```python
from build123d import *

# Parameters (mm, degrees)
SKETCH_1_W             = 160
SKETCH_1_H             = 124
EXTRUDE_1_DEPTH        = 3
SKETCH_2_R             = 1.5
CUT_EXTRUDE_1_DEPTH    = 10
SKETCH_3_R             = 2
CUT_EXTRUDE_2_DEPTH    = 172.618763543
SKETCH_4_R             = 1.5
CUT_EXTRUDE_3_DEPTH    = 10
PATTERN_LINEAR_1_COUNT = 7
PATTERN_LINEAR_1_PITCH = 8
SKETCH_6_R             = 1.5
CUT_EXTRUDE_4_DEPTH    = 10
SKETCH_7_R             = 1.5
CUT_EXTRUDE_5_DEPTH    = 10
SKETCH_8_R             = 1.5
CUT_EXTRUDE_6_DEPTH    = 10
SKETCH_9_R             = 1.5
CUT_EXTRUDE_7_DEPTH    = 10
SKETCH_10_R            = 4
CUT_EXTRUDE_8_DEPTH    = 10
FILLET_1_R             = 2
SKETCH_12_R            = 1.5
CUT_EXTRUDE_10_DEPTH   = 10
SKETCH_13_R            = 1.75
CUT_EXTRUDE_11_DEPTH   = 70
SKETCH_14_R            = 1.5
CUT_EXTRUDE_12_DEPTH   = 4
SKETCH_15_R            = 2.5
CUT_EXTRUDE_13_DEPTH   = 10


with BuildPart() as part:
    # 草圖1 → 填料-伸長1 (new body)
    with BuildSketch(Plane(origin=(0, 0, 0), x_dir=(1, 0, 0), z_dir=(0, 1, 0))):
        with Locations((80, 0)):
            Rectangle(SKETCH_1_W, SKETCH_1_H)
    extrude(amount=EXTRUDE_1_DEPTH)

    # 草圖2 → 除料-伸長1 (cut)
    with BuildSketch(Plane(origin=(0, 3, 0), x_dir=(1, 0, 0), z_dir=(0, 1, 0))):
        with Locations(Location((113, 52, 0), (0, 0, 270))):
            Circle(SKETCH_2_R)
        with Locations(Location((130, 52, 0), (0, 0, 270))):
            Circle(SKETCH_2_R)
        with Locations(Location((113, -52, 0), (0, 0, 270))):
            Circle(SKETCH_2_R)
        with Locations(Location((130, -52, 0), (0, 0, 270))):
            Circle(SKETCH_2_R)
    extrude(amount=-CUT_EXTRUDE_1_DEPTH, mode=Mode.SUBTRACT)

    # 草圖3 → 除料-伸長2 (cut, through all)
    with BuildSketch(Plane.XZ):
        with Locations(Location((25, 19.5, 0), (0, 0, 270))):
            Circle(SKETCH_3_R)
        with Locations(Location((25, -19.5, 0), (0, 0, 270))):
            Circle(SKETCH_3_R)
    extrude(amount=-CUT_EXTRUDE_2_DEPTH, mode=Mode.SUBTRACT)

    # 草圖4 → 除料-伸長3 (cut)
    with BuildSketch(Plane(origin=(0, 3, 0), x_dir=(1, 0, 0), z_dir=(0, 1, 0))):
        with Locations(Location((5, 24, 0), (0, 0, 270))):
            Circle(SKETCH_4_R)
    cut_extrude_3 = extrude(amount=-CUT_EXTRUDE_3_DEPTH, mode=Mode.SUBTRACT)

    # 直線複製排列1: 除料-伸長3 ×7
    with Locations(*[(0, 0, i * PATTERN_LINEAR_1_PITCH) for i in range(1, PATTERN_LINEAR_1_COUNT)]):
        add(cut_extrude_3, mode=Mode.SUBTRACT)

    # 草圖6 → 除料-伸長4 (cut)
    with BuildSketch(Plane(origin=(0, 3, 0), x_dir=(1, 0, 0), z_dir=(0, 1, 0))):
        with Locations(Location((100, 19, 0), (0, 0, 270))):
            Circle(SKETCH_6_R)
        with Locations(Location((137, 19, 0), (0, 0, 270))):
            Circle(SKETCH_6_R)
        with Locations(Location((100, -18, 0), (0, 0, 270))):
            Circle(SKETCH_6_R)
        with Locations(Location((137, -18, 0), (0, 0, 270))):
            Circle(SKETCH_6_R)
    extrude(amount=-CUT_EXTRUDE_4_DEPTH, mode=Mode.SUBTRACT)

    # 草圖7 → 除料-伸長5 (cut)
    with BuildSketch(Plane(origin=(0, 3, 0), x_dir=(1, 0, 0), z_dir=(0, 1, 0))):
        with Locations(Location((49.8, 30.6, 0), (0, 0, 270))):
            Circle(SKETCH_7_R)
        with Locations(Location((77.8, 30.6, 0), (0, 0, 270))):
            Circle(SKETCH_7_R)
        with Locations(Location((34.6, -20.4, 0), (0, 0, 270))):
            Circle(SKETCH_7_R)
        with Locations(Location((82.6, -21, 0), (0, 0, 270))):
            Circle(SKETCH_7_R)
    extrude(amount=-CUT_EXTRUDE_5_DEPTH, mode=Mode.SUBTRACT)

    # 草圖8 → 除料-伸長6 (cut)
    with BuildSketch(Plane(origin=(0, 3, 0), x_dir=(1, 0, 0), z_dir=(0, 1, 0))):
        with Locations(Location((37, 52, 0), (0, 0, 270))):
            Circle(SKETCH_8_R)
        with Locations(Location((145, 52, 0), (0, 0, 270))):
            Circle(SKETCH_8_R)
        with Locations(Location((37, -52, 0), (0, 0, 270))):
            Circle(SKETCH_8_R)
        with Locations(Location((145, -52, 0), (0, 0, 270))):
            Circle(SKETCH_8_R)
    extrude(amount=-CUT_EXTRUDE_6_DEPTH, mode=Mode.SUBTRACT)

    # 草圖9 → 除料-伸長7 (cut)
    with BuildSketch(Plane(origin=(0, 3, 0), x_dir=(1, 0, 0), z_dir=(0, 1, 0))):
        with Locations(Location((91, -52, 0), (0, 0, 270))):
            Circle(SKETCH_9_R)
        with Locations(Location((91, 52, 0), (0, 0, 270))):
            Circle(SKETCH_9_R)
    extrude(amount=-CUT_EXTRUDE_7_DEPTH, mode=Mode.SUBTRACT)

    # 草圖10 → 除料-伸長8 (cut)
    with BuildSketch(Plane(origin=(0, 3, 0), x_dir=(1, 0, 0), z_dir=(0, 1, 0))):
        with Locations(Location((25, 37, 0), (0, 0, 270))):
            Circle(SKETCH_10_R)
        with Locations(Location((25, -37, 0), (0, 0, 270))):
            Circle(SKETCH_10_R)
    extrude(amount=-CUT_EXTRUDE_8_DEPTH, mode=Mode.SUBTRACT)

    # 圓角1
    fillet_1_edges = [part.edges().sort_by_distance(p)[0] for p in [
        (160, 1.5, -62),
        (160, 1.5, 62),
    ]]
    fillet(fillet_1_edges, radius=FILLET_1_R)

    # 草圖12 → 除料-伸長10 (cut)
    with BuildSketch(Plane.XZ):
        with Locations(Location((65, 40, 0), (0, 0, 270))):
            Circle(SKETCH_12_R)
        with Locations(Location((115, 40, 0), (0, 0, 270))):
            Circle(SKETCH_12_R)
        with Locations(Location((65, -40, 0), (0, 0, 270))):
            Circle(SKETCH_12_R)
        with Locations(Location((115, -40, 0), (0, 0, 270))):
            Circle(SKETCH_12_R)
    extrude(amount=-CUT_EXTRUDE_10_DEPTH, mode=Mode.SUBTRACT)

    # 草圖13 → 除料-伸長11 (cut)
    with BuildSketch(Plane.XZ):
        with Locations(Location((8.5, 53.5, 0), (0, 0, 270))):
            Circle(SKETCH_13_R)
        with Locations(Location((17.1, 29.2, 0), (0, 0, 270))):
            Circle(SKETCH_13_R)
    extrude(amount=-CUT_EXTRUDE_11_DEPTH, mode=Mode.SUBTRACT)

    # 草圖14 → 除料-伸長12 (cut)
    with BuildSketch(Plane.XZ):
        with Locations(Location((54.05, -55, 0), (0, 0, 270))):
            Circle(SKETCH_14_R)
        with Locations(Location((45.75, -55, 0), (0, 0, 270))):
            Circle(SKETCH_14_R)
    extrude(amount=-CUT_EXTRUDE_12_DEPTH, mode=Mode.SUBTRACT)

    # 草圖15 → 除料-伸長13 (cut)
    with BuildSketch(Plane.XZ):
        with Locations(Location((90, 35, 0), (0, 0, 270))):
            Circle(SKETCH_15_R)
    extrude(amount=-CUT_EXTRUDE_13_DEPTH, mode=Mode.SUBTRACT)


solid = part.part
```
Design review of the part built by this model. Coordinates are the model's own, in mm. Coordinates: 2 decimals unless noted, no trailing zeros. Write each loop counter-clockwise with the first axis right and the second up, starting at its lowest first coordinate (ties: lowest second). Pieces come first, ordered by that corner, then holes.
1) To check wall thickness, follow L1, parallel to Z at x = 137, y = 2.3; L2, parallel to Z at x = 113, y = 0.65; L3, parallel to X at y = 2.1, z = 36. State the ranges of each line that lie inside material, in increasing order.
2) Mouldability with a two-part tool opening along Z and no side actions: class faces 1 (the flat face through (79, 0, -1)), 2 (the cylindrical face through (23.226, 1.479, 18.577)) as +Z half, -Z half, draft (parallel to the pull), parting line (faces both ways), or undercut.
3) Add section B-B (y = 1.1). State how many separate pieces and enclosed holes the cut face has, plus the area to 3 significant figures.
4) Add section A-A (x = 8.5). Write out the cut boundary in (y, z), plus the area to 4 significant figures.
Check result:
1. L1: z = -62 to -20.5, -17.5 to 16.5, 19.5 to 62
1. L2: z = -62 to -53.5, -50.5 to 50.5, 53.5 to 62
1. L3: x = 0 to 21.13, 28.87 to 87.71, 92.29 to 160
2. face 1: draft
2. face 2: undercut
3. separate pieces: 1
3. enclosed holes: 38
3. area: 19,500 mm2
4. outline: (0, -62) - (3, -62) - (3, 51.75) - (0, 51.75) - close; (0, 55.25) - (3, 55.25) - (3, 62) - (0, 62) - close
4. area: 361.5 mm2
